Part print with two shaded views. Sizes in mm from the minimum x, y, z corner. A direction names the side the tool comes from. Round coordinates to 2 decimals unless told otherwise and drop trailing zeros. Loops run counter-clockwise (first coordinate to the right, second up) from the corner with the lowest first, then second, coordinate; pieces in that order, holes last. Notation, with made-up numbers: (5, 35.25) - (14, 35.25) arc R27 cw to (14, 67.25) - close; hole circle Ø1 at (75, -33.5). An arc over 180 degrees is marked (long way). Use a Markdown table: item, result.
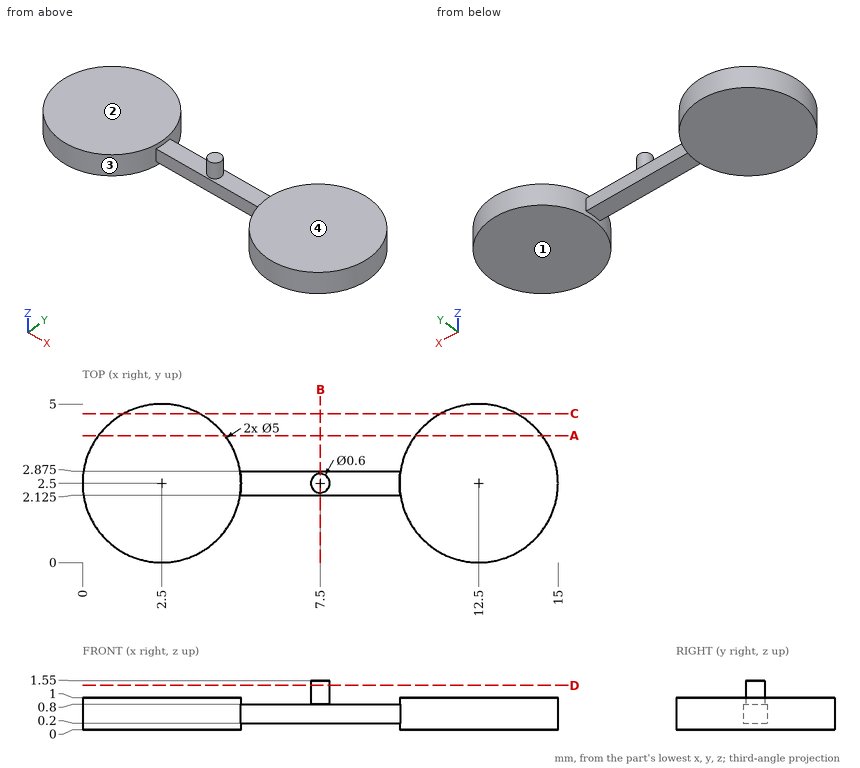
Q1. Pull direction X, two halves, no side cores. Call the marked faces 3 and 4: pulls with the +X half, pulls with the -X half, needs draft (parallel to the pull), parting line crosses it, or undercut.
Results found:
| item | result |
|---|---|
| face 3 | undercut |
| face 4 | needs draft |
Q2. Cut at D-D, the plane z = 1.4. List the corners of the cut face in (x, y).
Results found:
| item | result |
|---|---|
| outline | circle Ø0.6 at (7.5, 2.5) |
Q3. Cut at C-C, the plane y = 4.7. List the corners of the cut face in (x, z).
Results found:
| item | result |
|---|---|
| outline | (1.31, 0) - (3.69, 0) - (3.69, 1) - (1.31, 1) - close; (11.31, 0) - (13.69, 0) - (13.69, 1) - (11.31, 1) - close |
Q4. Drop flat-ended pins along their axis: pin 1 (3 mm diameter, centred on x = 8.5, y = 0.5, fed in from +Z); pin 2 (0.7 mm diameter, centred on x = 6.5, z = 0.5, fed in from -Y) (3 decimals); pin 3 (1.5 mm diameter, centred on x = 1.5, y = 1.5, fed in from +Z); pin 4 (0.5 mm diameter, centred on x = 7.5, z = 0.5, fed in from +Y) (3 decimals). Give the stop position or say it passes through.
Results found:
| item | result |
|---|---|
| pin 1 | passes through |
| pin 2 | stops at y = 2.125 |
| pin 3 | stops at z = 1 |
| pin 4 | stops at y = 2.875 |
Q5. Cut at B-B, the plane x = 7.5. List the corners of the cut face in (y, z) (3 decimals).
Results found:
| item | result |
|---|---|
| outline | (2.125, 0.2) - (2.875, 0.2) - (2.875, 0.8) - (2.8, 0.8) - (2.8, 1.55) - (2.2, 1.55) - (2.2, 0.8) - (2.125, 0.8) - close |
Q6. Which spindle directions (+Z, -Z, +X, -X, +Y, -Y) get a long thin tool onto all of the face, cutting with end or side? Do the marked faces 1 and 2. Say none if no direction does.
Results found:
| item | result |
|---|---|
| face 1 | -Z, +X, -X, +Y, -Y |
| face 2 | +Z, -X, +Y, -Y |
Q7. Cut at A-A, the plane y = 4. List the corners of the cut face in (x, z), plus the area to 3 significant figures.
Results found:
| item | result |
|---|---|
| outline | (0.5, 0) - (4.5, 0) - (4.5, 1) - (0.5, 1) - close; (10.5, 0) - (14.5, 0) - (14.5, 1) - (10.5, 1) - close |
| area | 8.00 mm2 |
Q8. Probe line 1 (Y direction, x = 7, z = 0.55) (3 decimals); line 2 (X direction, y = 0.3, z = 0.1); line 3 (X direction, y = 0.75, z = 0.4). List the from-to ranges inside material, lowest first.
Results found:
| item | result |
|---|---|
| line 1 | y = 2.125 to 2.875 |
| line 2 | x = 1.31 to 3.69, 11.31 to 13.69 |
| line 3 | x = 0.71 to 4.29, 10.71 to 14.29 |
